Design review of the part built by this model. Coordinates are the model's own, in mm. A direction names the side the tool comes from. Round coordinates to 2 decimals unless told otherwise and drop trailing zeros. Write each loop counter-clockwise with the first axis right and the second up, starting at its lowest first coordinate (ties: lowest second). Pieces come first, ordered by that corner, then holes. Notation, with made-up numbers: (5.5, 70) -> (16.5, 70) arc R7 ccw to (16.5, 78) -> close; hole circle Ø5 at (12.25, 54.5). An arc over 180 degrees is marked (long way). Write item = value, one per line. Start each with the question number.
Item 1: Machinability: for faces 5 (the flat face through (10, 2.3, 4)), 6 (the flat face through (9, -5, 4)), 7 (the flat face through (5.4, -6.1, -0.6)), 8 (the cylindrical face through (6, 0, 2.5)), 9 (the cylindrical face through (4.121, -2.253, -4.945)), which of the approach directions +Z, -Z, +X, -X, +Y, -Y give a long, thin tool a straight path to every point of the face, cutting with its end or side? Answer none if there is none.
Item 2: To check wall thickness, follow L1, parallel to X at y = -5, z = -2.2; L2, parallel to X at y = 5.5, z = -3.25; L3, parallel to Y at x = 4, z = 3.5. State the ranges of each line that lie inside material, in increasing order.
Item 3: Add section C-C, the plane x = 4. State how many separate pieces and enclosed holes the cut face has, then the cut area to 3 significant figures.
Item 4: Add section A-A, the plane x = 10. State the section outline as (y, z) points, then the cut area to 3 significant figures.
Item 5: Add section B-B, the plane y = 0. State the section outline as (x, z) points, then the cut area to 3 significant figures.
Item 6: Mouldability with a two-part tool opening along Y and no side actions: class faces 1 (the flat face through (10, 2.3, -5)), 2 (the flat face through (10, -2.3, 5)), 3 (the flat face through (2.8, -6.2, -3)), 4 (the flat face through (0, 2, 2)) as released by +Y, released by -Y, zero draft, split by the parting line, or undercut.
Item 7: For pin 1 Ø2.5 at (x, z) = (10, 3.5) entering from -Y; pin 2 Ø5 at (x, y) = (6.5, -6) entering from -Z; pin 3 Ø4 at (x, y) = (4, 4) entering from -Z, all flat-tipped, find the tip position at first contact; note any pin that passes through.
Autodesk Inventor part; units mm, degrees
ref_plane "L_XY" through (12.2, 0, 0) normal (1, 0, 0) x (0, 0, -1)
ref_plane "L_YZ" through (12.2, 0, 0) normal (0, 0, -1) x (0, 1, 0)
ref_plane "L_ZX" through (12.2, 0, 0) normal (0, 1, 0) x (1, 0, 0)
sketch "Sketch_1" plane through (0, 0, 0) normal (0, 0, 1) x (1, 0, 0)
  line L0 (11.9, 0) -> (0, 0)
  line L1 (0, 0) -> (0, 8.2)
  line L2 (0, 8.2) -> (0.2, 8.4)
  line L3 (0.2, 8.4) -> (11.9, 8.4)
  line L4 (11.9, 8.4) -> (11.9, 0)
  line L5 (11.9, 0) -> (0, 0)
revolve "Revolution1" add sketch "Sketch_1" angle 360 about axis through (11.9, 0, 0) along (1, 0, 0)
sketch "Sketch_6" plane through (0, 0, 0) normal (1, 0, 0) x (0, 1, 0)
  line L0 (0, 0.6) -> (-8.4, 0.6)
  line L1 (-8.4, 0.6) -> (-8.4, -0.6)
  line L2 (-8.4, -0.6) -> (0, -0.6)
  line L3 (0, -0.6) -> (0, 0.6)
extrude "Extrusion1" cut sketch "Sketch_6" along normal blind 9
sketch "Sketch_7" plane through (4, 0, 0) normal (1, 0, 0) x (0, 0, -1)
  line L0 (-8.4, -5) -> (8.4, -5)
  line L1 (8.4, -5) -> (8.4, -7.75)
  line L2 (8.4, -7.75) -> (3, -7.75)
  line L3 (3, -7.75) -> (3, -6.5)
  line L4 (3, -6.5) -> (0.6, -6.5)
  line L5 (0.6, -6.5) -> (0.6, -5)
  line L6 (0.6, -5) -> (8.4, -5)
revolve "Revolution2" cut sketch "Sketch_7" angle 360 about axis through (4, -5, 8.4) along (0, 0, 1)
sketch "Sketch_13" plane through (4, 0, 0) normal (1, 0, 0) x (0, 0, -1)
  line L0 (-8.4, -5) -> (8.4, -5)
  line L1 (-0.6, -5) -> (-0.6, -6.2295)
  line L2 (-0.6, -6.2295) -> (-8.4, -6.2295)
  line L3 (-8.4, -6.2295) -> (-8.4, -5)
  line L4 (-8.4, -5) -> (-0.6, -5)
revolve "Revolution3" cut sketch "Sketch_13" angle 360 about axis through (4, -5, 8.4) along (0, 0, 1)
thread "Thread1"
sketch "Sketch_2" plane through (11.9, 0, 0) normal (1, 0, 0) x (0, 0, -1)
  line L0 (-9.4, 8.9) -> (-9.4, -8.9)
  line L1 (-9.4, -8.9) -> (9.4, -8.9)
  line L2 (9.4, -8.9) -> (9.4, 8.9)
  line L3 (9.4, 8.9) -> (-9.4, 8.9)
  line L4 (-8.4, 2.3) -> (-8.4, -2.3)
  line L5 (-8.4, -2.3) -> (8.4, -2.3)
  line L6 (8.4, -2.3) -> (8.4, 2.3)
  line L7 (8.4, 2.3) -> (-8.4, 2.3)
extrude "Extrusion2" cut sketch "Sketch_2" against normal blind 2.9
sketch "Sketch_3" plane through (0, 0, 0) normal (0, 0, 1) x (1, 0, 0)
  line L0 (11.9, 0) -> (0, 0)
  line L1 (0, 0) -> (0, 2.5)
  line L2 (0, 2.5) -> (11.9, 2.5)
  line L3 (11.9, 2.5) -> (11.9, 0)
  line L4 (11.9, 0) -> (0, 0)
revolve "Revolution4" cut sketch "Sketch_3" angle 360 about axis through (11.9, 0, 0) along (1, 0, 0)
sketch "Sketch_17" plane through (0, 0, 0) normal (1, 0, 0) x (0, 0, -1)
  line L0 (-0.6, 0) -> (0.6, 0)
  line L1 (0.6, 0) -> (0.6, 4.44)
  line L2 (0.6, 4.44) -> (-0.6, 4.44)
  line L3 (-0.6, 4.44) -> (-0.6, 0)
extrude "Extrusion3" cut sketch "Sketch_17" along normal blind 11.9
ref_plane "L_XY" through (12.2, 0, 0) normal (1, 0, 0) x (0, 0, -1)
ref_plane "L_YZ" through (12.2, 0, 0) normal (0, 0, -1) x (0, 1, 0)
ref_plane "L_ZX" through (12.2, 0, 0) normal (0, 1, 0) x (1, 0, 0)
ref_plane "screw_XY" through (4, -5, -3) normal (0, 0, -1) x (1, 0, 0)
ref_plane "screw_YZ" through (4, -5, -3) normal (1, 0, 0) x (0, -1, 0)
ref_plane "screw_ZX" through (4, -5, -3) normal (0, -1, 0) x (0, 0, -1)
properties part number "MCOC17-5_c"
Result set:
q1.face_5 = +Z, -Z, +X, +Y
q1.face_6 = +Z, -Z, +X, -Y
q1.face_7 = +X, -X, -Y
q1.face_8 = +X, -X
q1.face_9 = -Z
q2.L1 = 0 to 2.5, 5.5 to 9
q2.L2 = 0 to 9
q2.L3 = -7.64 to -6.23, -3.77 to 7.64
q3.separate_pieces = 3
q3.enclosed_holes = 0
q3.area = 152 mm²
q4.outline = (-2.3, -8.08) arc R8.4 ccw to (2.3, -8.08) -> (2.3, -0.98) arc R2.5 cw to (-2.3, -0.98) -> close; (-2.3, 0.98) arc R2.5 cw to (2.3, 0.98) -> (2.3, 8.08) arc R8.4 ccw to (-2.3, 8.08) -> close
q4.area = 57.2 mm²
q5.outline = (0, -8.2) -> (0.2, -8.4) -> (11.9, -8.4) -> (11.9, -2.5) -> (0, -2.5) -> close; (0, 2.5) -> (11.9, 2.5) -> (11.9, 8.4) -> (0.2, 8.4) -> (0, 8.2) -> close
q5.area = 140 mm²
q6.face_1 = released by +Y
q6.face_2 = released by -Y
q6.face_3 = undercut
q6.face_4 = zero draft
q7.pin_1 = -7.94
q7.pin_2 = -7.64
q7.pin_3 = -8.16
